Work out the finished part from the listing and answer in its coordinate system (mm). Face numbers are marked on the shaded views. A direction names the side the tool comes from. Round coordinates to 2 decimals unless told otherwise and drop trailing zeros. Order: outer loops, then holes, each group sorted by start corner. A loop starts at its lowest first (then second) coordinate and runs counter-clockwise, first axis right, second up. Notation, with made-up numbers: (76, 5.5) - (114, 5.5) arc R20 ccw to (114, 33.5) - close; hole circle Ø8 at (57.5, 27). An arc over 180 degrees is marked (long way). Use one line per item in the form item = value. Start each with the question number.
Q1. Which of the six approach directions +Z, -Z, +X, -X, +Y, -Y give full straight-line access (tool end or side, diameter ignored) to the marked faces 4 and 5?
Q2. Given P1, Ø1, axis at x = 4, z = 10.5, coming from the +Y side; P2, Ø12, axis at x = 18, y = -10, coming from the +Z side; P3, Ø3, axis at x = -13.5, z = 10, coming from the +Y side; P4, Ø11, axis at y = -8, z = 8, coming from the -X side, each flat-ended and moving along its own axis, determine where each tip first touches the part or whether it passes through.
Q3. The part is cut by section A-A on x = -9.5. Determine the outline of the cut face in (y, z) (1 decimal).
Q4. For a pull along X with two mould halves and no side action, classify the marked faces 1, 2 and 3 as +X half, -X half, draft (parallel to the pull), parting line (faces both ways), or undercut.
Q5. Find the intervals of material crossed by line 1 (Z direction, x = -8.5, y = 0); line 2 (Z direction, x = -10.5, y = 4); line 3 (X direction, y = -14.5, z = -13), in increasing order. Write a range as [from, to].
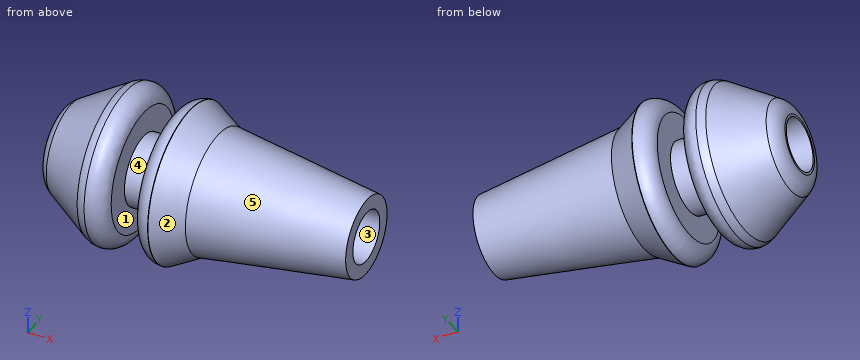
from build123d import *

# Parameters (mm, degrees)
F2_F1_R  = 6.35
F2_F2_R  = 6.35
F3_R     = 7.9375
F4_DEPTH = 93.7661007047
F6_R     = 5.08


# Not quite as in the source:
# - two fillets or chamfers of one size are made in one step


with BuildPart() as f1:
    # F0 (on Top) → F1 (revolve)
    with BuildSketch(Plane.XY):
        Polygon((-39.1627885401, 12.2120529413), (-39.1627885401, 0), (54.6033121645, 0), (54.6033121645, 12.2120529413), (8.8432114571, 18.6689998955), (0, 23.7222649157), (-5.1936330274, 23.7222649157), (-5.1936330274, 10.8083682135), (-13.8964727521, 10.8083682135), (-13.8964727521, 23.7222649157), (-20.6341594458, 23.7222649157), align=None)
    revolve(axis=Axis((7.7202618122, 0, 0), (1, 0, 0)))

    # F2: fillet of radius 6.35 on 2 edges, made by hand

    # F2_f1
    f2_f1_edges = [f1.edges().sort_by_distance(p)[0] for p in [
        (-39.1627885401, -12.2120529413, 0),
    ]]
    fillet(f2_f1_edges, radius=F2_F1_R)

    # F2_f2
    f2_f2_edges = [f1.edges().sort_by_distance(p)[0] for p in [
        (-20.6341594458, -23.7222649157, 0),
    ]]
    fillet(f2_f2_edges, radius=F2_F2_R)

    # F3 (on face) → F4 (cut, through all)
    with BuildSketch(Plane.YZ.offset(54.6033121645)):
        Circle(F3_R)
    extrude(amount=-F4_DEPTH, mode=Mode.SUBTRACT)

    # F6
    f6_edges = [f1.edges().sort_by_distance(p)[0] for p in [
        (-13.896473, -23.722265, 0),
        (-5.193633, -23.722265, 0),
    ]]
    fillet(f6_edges, radius=F6_R)


solid = f1.part
Found:
q1.face_4 = none
q1.face_5 = +X
q2.P1 = 19.11
q2.P2 = 17.14
q2.P3 = 19.49
q2.P4 = -39.16
q3.outline = circle Ø21.6 at (0, 0); hole circle Ø15.9 at (0, 0)
q4.face_1 = undercut
q4.face_2 = +X half
q4.face_3 = draft
q5.line_1 = [-10.81, -7.94], [7.94, 10.81]
q5.line_2 = [-10.04, -6.86], [6.86, 10.04]
q5.line_3 = [-27.47, -13.97], [-5.13, 7.43]
